The listing builds one solid part. Answer for the finished solid, in the listing's coordinates (mm). A direction names the side the tool comes from. Round coordinates to 2 decimals unless told otherwise and drop trailing zeros. Loops run counter-clockwise (first coordinate to the right, second up) from the corner with the lowest first, then second, coordinate; pieces in that order, holes last. Notation, with made-up numbers: (-35.75, -14) -> (-21.75, -14) arc R30 ccw to (-21.75, 20) -> close; hole circle Ø7 at (-6.5, 48). An arc over 180 degrees is marked (long way). Write each question's results on one line, items separated by ' | '. Start each with the question number.
from build123d import *

# Parameters (mm, degrees)
SKETCH1_R           = 2
SKETCH1_W           = 5.1
SKETCH1_H           = 5.1
BOSS_EXTRUDE1_DEPTH = 5
CONG_2_R            = 3


with BuildPart() as part:
    # Sketch1 → Boss-Extrude1 (new body)
    with BuildSketch(Plane.XY):
        with BuildLine():
            Line((24.248711306, 2.5), (13.520817283, 2.5))
            ThreePointArc((13.520817283, 2.5), (-13.75, 0), (13.520817283, -2.5))
            Line((13.520817283, -2.5), (24.248711306, -2.5))
            Line((24.248711306, -2.5), (24.248711306, -42))
            Line((24.248711306, -42), (-48.497422612, 0))
            Line((-48.497422612, 0), (24.248711306, 42))
            Line((24.248711306, 42), (24.248711306, 2.5))
        make_face()
        with Locations((14, 24.248711306)):
            Circle(SKETCH1_R, mode=Mode.SUBTRACT)
        with Locations((14, -24.248711306)):
            Circle(SKETCH1_R, mode=Mode.SUBTRACT)
        with Locations((-28, 0)):
            Circle(SKETCH1_R, mode=Mode.SUBTRACT)
        with Locations((0, 20.5)):
            Rectangle(SKETCH1_W, SKETCH1_H, mode=Mode.SUBTRACT)
        Polygon((21.236885557, 9.31663522), (16.820155998, 6.76663522), (14.270155998, 11.18336478), (18.686885557, 13.73336478), align=None, mode=Mode.SUBTRACT)
        Polygon((18.686885557, -13.73336478), (14.270155998, -11.18336478), (16.820155998, -6.76663522), (21.236885557, -9.31663522), align=None, mode=Mode.SUBTRACT)
        with Locations((0, -20.5)):
            Rectangle(SKETCH1_W, SKETCH1_H, mode=Mode.SUBTRACT)
        Polygon((-21.236885557, -9.31663522), (-16.820155998, -6.76663522), (-14.270155998, -11.18336478), (-18.686885557, -13.73336478), align=None, mode=Mode.SUBTRACT)
        Polygon((-18.686885557, 13.73336478), (-14.270155998, 11.18336478), (-16.820155998, 6.76663522), (-21.236885557, 9.31663522), align=None, mode=Mode.SUBTRACT)
    extrude(amount=BOSS_EXTRUDE1_DEPTH)

    # Congé2
    cong_2_edges = [part.edges().sort_by_distance(p)[0] for p in [
        (24.248711306, 2.5, 2.5),
        (13.520817283, 2.5, 2.5),
        (13.520817283, -2.5, 2.5),
        (24.248711306, -2.5, 2.5),
    ]]
    fillet(cong_2_edges, radius=CONG_2_R)


solid = part.part
Item 1: The part is cut by section D-D, the plane y = 32.5. Give the vertices of the cut face in (x, z).
Item 2: The part is cut by section B-B, the plane x = 0. Give the vertices of the cut face in (y, z).
Item 3: For faces 4 (the flat face through (24.249, 24, 2)), 5 (the cylindrical face through (23.35, 3.36, 2.54)), 6 (the flat face through (-19.06, -8.06, 2.46)), determine the directions among +Z, -Z, +X, -X, +Y, -Y from which every point of the face is accessible in a straight line to the end or side of a thin tool.
Item 4: Determine the mould class of faces 1 (the flat face through (24.249, -23, 2)), 2 (the flat face through (-2.55, -21, 2)), 3 (the flat face through (-11.62, -21.29, 2.46)) for opening direction Y: +Y half, -Y half, draft (parallel to the pull), parting line (faces both ways), or undercut.
Item 5: The part is cut by section A-A, the plane x = -28. Give the vertices of the cut face in (y, z), plus the area to 3 significant figures.
Item 6: The part is cut by section C-C, the plane z = 4.05. Give the number of separate pieces and of enclosed holes in the cut face, plus the area to 3 significant figures.
Item 7: Each of these flat-tipped pins is pushed along its axis until it touches: pin 1 Ø2 at (y, z) = (-4.5, 1) entering from +X; pin 2 Ø2.5 at (y, z) = (-20, 3) entering from -X; pin 3 Ø1.5 at (x, z) = (0, 2.5) entering from +Y; pin 4 Ø2.5 at (y, z) = (21, 1.5) entering from -X. Where does it stop, or does it pass through?
Item 8: Straight lines are drawn through the part: L1, parallel to Y at x = 14, z = 3.05; L2, parallel to Y at x = 0, z = 2.95; L3, parallel to X at y = -0.5, z = 3.35. For each, find the intervals that lie inside material, in ascending order. Write a range as [from, to].
Report:
1) outline: (7.79, 0) -> (24.25, 0) -> (24.25, 5) -> (7.79, 5) -> close
2) outline: (-28, 0) -> (-23.05, 0) -> (-23.05, 5) -> (-28, 5) -> close; (-17.95, 0) -> (-13.75, 0) -> (-13.75, 5) -> (-17.95, 5) -> close; (13.75, 0) -> (17.95, 0) -> (17.95, 5) -> (13.75, 5) -> close; (23.05, 0) -> (28, 0) -> (28, 5) -> (23.05, 5) -> close
3) face 4: +Z, -Z, +X, +Y, -Y | face 5: +Z, -Z, +X | face 6: +Z, -Z
4) face 1: draft | face 2: undercut | face 3: -Y half
5) outline: (-11.83, 0) -> (-2, 0) -> (-2, 5) -> (-11.83, 5) -> close; (2, 0) -> (11.83, 0) -> (11.83, 5) -> (2, 5) -> close | area: 98.3 mm2
6) separate pieces: 1 | enclosed holes: 9 | area: 2,210 mm2
7) pin 1: stops at x = 24.25 | pin 2: stops at x = -16.02 | pin 3: stops at y = 28.43 | pin 4: stops at x = -14.29
8) L1: y = [-36.08, -26.25], [-22.25, -3.12], [3.12, 22.25], [26.25, 36.08] | L2: y = [-28, -23.05], [-17.95, -13.75], [13.75, 17.95], [23.05, 28] | L3: x = [-47.63, -29.94], [-26.06, -13.74]
